Geometry check sheet. Reference: drawing and pictorial views, mm from the part's lowest x, y, z. Give positions to 0.01 mm unless a question says otherwise; leave off trailing zeros. Loops run counter-clockwise (first coordinate to the right, second up) from the corner with the lowest first, then second, coordinate; pieces in that order, holes last. Notation, with made-up numbers: (-11.5, -24.5) - (-1.5, -24.5) arc R20 ccw to (-1.5, -15.5) - close; hole circle Ø1 at (16, -13). An arc over 180 degrees is marked (long way). Use CSV: the item, a comma, the result in double quotes.
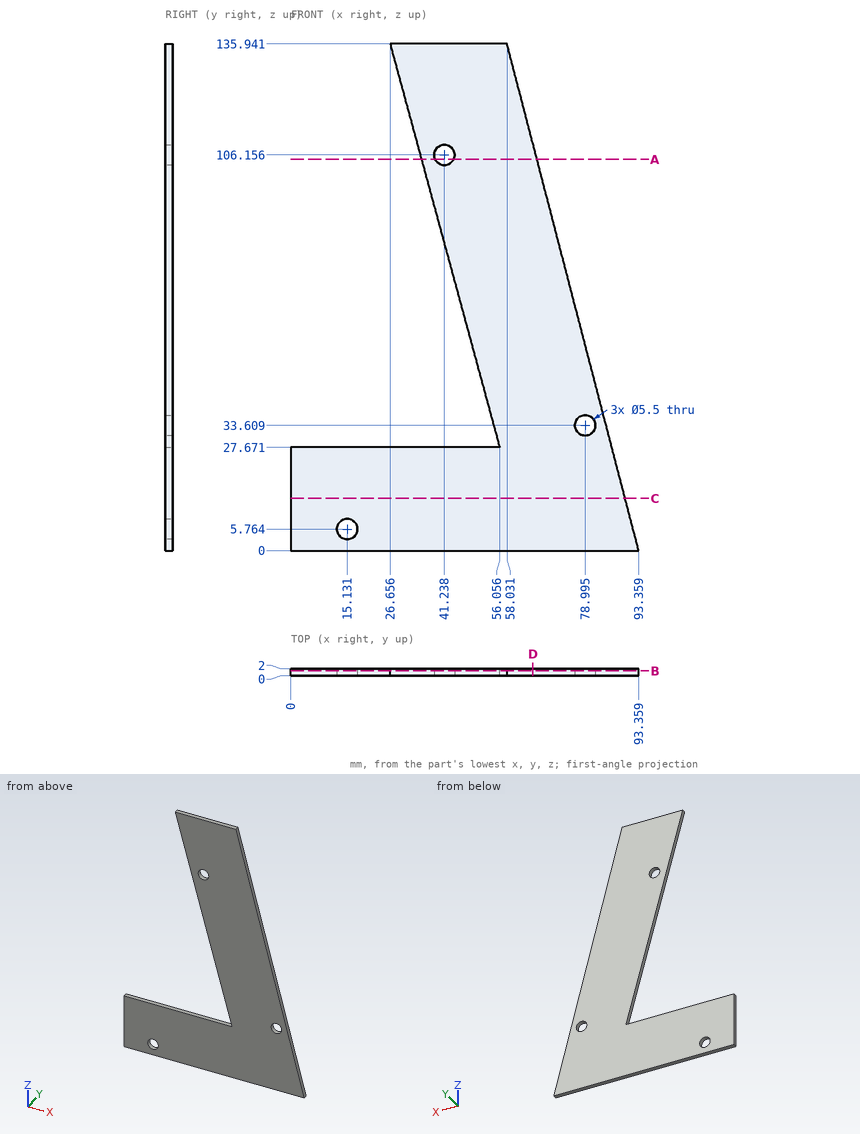
1. Go/stop test with a flat-tipped pin: pin 1 Ø1 at (x, y) = (17, 1.5) entering from +Z. Record where the tip stops, or that it passes through.
Completed:
pin 1,"stops at z = 27.67"
2. Sectioned sample at D-D, the plane x = 65. Record the boundary of the cut face in (y, z).
Completed:
outline,"(0, 0) - (2, 0) - (2, 109.13) - (0, 109.13) - close"
3. Scan lines: line 1 along Z through (x, y) = (9, 0.55); line 2 along Z through (x, y) = (13, 0.1) (1 decimal); line 3 along X through (y, z) = (0.2, 6). Record each from-to range of solid material in increasing order.
Completed:
line 1,"z = 0 to 27.67"
line 2,"z = 0 to 4, 7.5 to 27.7"
line 3,"x = 0 to 12.39, 17.87 to 91.8"
4. Sectioned sample at B-B, the plane y = 1.4. State how many separate pieces and enclosed holes the cut face has, and give its area (3 significant figures).
Completed:
separate pieces,"1"
enclosed holes,"3"
area,"5,740 mm²"
5. Sectioned sample at A-A, the plane z = 105. Record the boundary of the cut face in (x, y).
Completed:
outline,"(35.06, 0) - (38.74, 0) - (38.74, 2) - (35.06, 2) - close; (43.73, 0) - (66.07, 0) - (66.07, 2) - (43.73, 2) - close"
6. Sectioned sample at C-C, the plane z = 14. Record the boundary of the cut face in (x, y).
Completed:
outline,"(0, 0) - (89.72, 0) - (89.72, 2) - (0, 2) - close"
